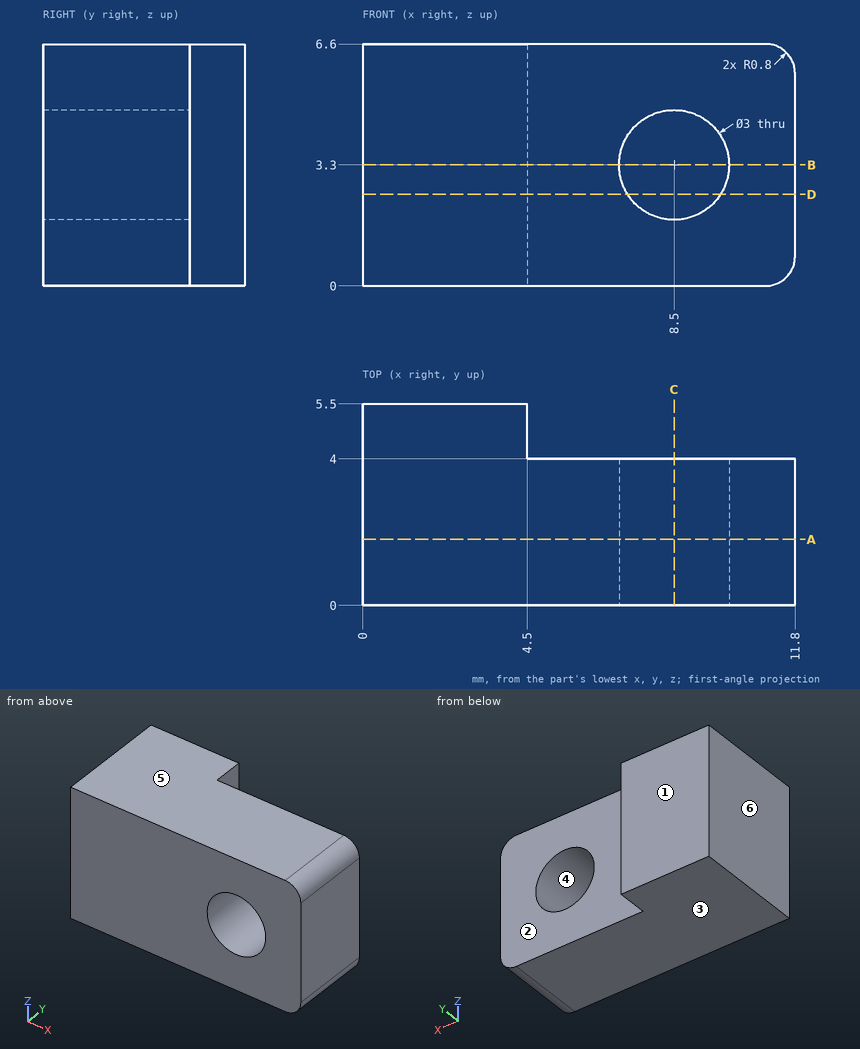
Source: three-view drawing plus pictorial views. Frame: mm from the lowest corner of the part. A direction names the side the tool comes from. Coordinates: 2 decimals unless noted, no trailing zeros. Order: outer loops, then holes, each group sorted by start corner. A loop starts at its lowest first (then second) coordinate and runs counter-clockwise, first axis right, second up. Notation, with made-up numbers: M 78,65.5 L 101,65.5 A23 cw 101,85.5 Z; hole C -36,-17.5 d3. An arc over 180 degrees is marked long. Answer in a Markdown table with one row per item.
(1) Section query B-B, the plane z = 3.3. Output: boundary loops of the cut face in (x, y), plus the area to 4 significant figures.
Numbers:
| item | result |
|---|---|
| outline | M 0,0 L 7,0 L 7,4 L 4.5,4 L 4.5,5.5 L 0,5.5 Z; M 10,0 L 11.8,0 L 11.8,4 L 10,4 Z |
| area | 41.95 mm^2 |
(2) Material intervals for line 1 (X direction, y = 2.6, z = 3.3); line 2 (X direction, y = 5.2, z = 2); line 3 (Y direction, x = 5.5, z = 1), sorted ascending. Write a range as [from, to].
Numbers:
| item | result |
|---|---|
| line 1 | x = [0, 7], [10, 11.8] |
| line 2 | x = [0, 4.5] |
| line 3 | y = [0, 4] |
(3) Section query C-C, the plane x = 8.5. Output: boundary loops of the cut face in (y, z).
Numbers:
| item | result |
|---|---|
| outline | M 0,0 L 4,0 L 4,1.8 L 0,1.8 Z; M 0,4.8 L 4,4.8 L 4,6.6 L 0,6.6 Z |
(4) Draft query along Z for the marked faces 3, 4, 5 and 6. Return one class per face: pulls with the +Z half, pulls with the -Z half, needs draft (parallel to the pull), parting line crosses it, or undercut.
Numbers:
| item | result |
|---|---|
| face 3 | pulls with the -Z half |
| face 4 | undercut |
| face 5 | pulls with the +Z half |
| face 6 | needs draft |
(5) Section query D-D, the plane z = 2.5. Output: boundary loops of the cut face in (x, y), plus the area to 3 significant figures.
Numbers:
| item | result |
|---|---|
| outline | M 0,0 L 7.23,0 L 7.23,4 L 4.5,4 L 4.5,5.5 L 0,5.5 Z; M 9.77,0 L 11.8,0 L 11.8,4 L 9.77,4 Z |
| area | 43.8 mm^2 |
(6) Section query A-A, the plane y = 1.8. Output: boundary loops of the cut face in (x, z), plus the area to 3 significant figures.
Numbers:
| item | result |
|---|---|
| outline | M 0,0 L 11,0 A0.8 ccw 11.8,0.8 L 11.8,5.8 A0.8 ccw 11,6.6 L 0,6.6 Z; hole C 8.5,3.3 d3 |
| area | 70.5 mm^2 |
(7) Contact query for flat-ended pins moving along their axis: pin 1 Ø3 at (x, z) = (6.5, 2.5) entering from +Y; pin 2 Ø1.2 at (y, z) = (4.5, 3) entering from +X. Output: stop coordinate, or through.
Numbers:
| item | result |
|---|---|
| pin 1 | stops at y = 4 |
| pin 2 | stops at x = 11.8 |
(8) Access query for the marked faces 1 and 2. Directions: +Z, -Z, +X, -X, +Y, -Y. A direction counts if a zero-diameter tool reaches every point of the face in a straight line with its end or side. Return the directions, or none.
Numbers:
| item | result |
|---|---|
| face 1 | +Z, -Z, +X, -X, +Y |
| face 2 | +Z, -Z, +X, +Y |
